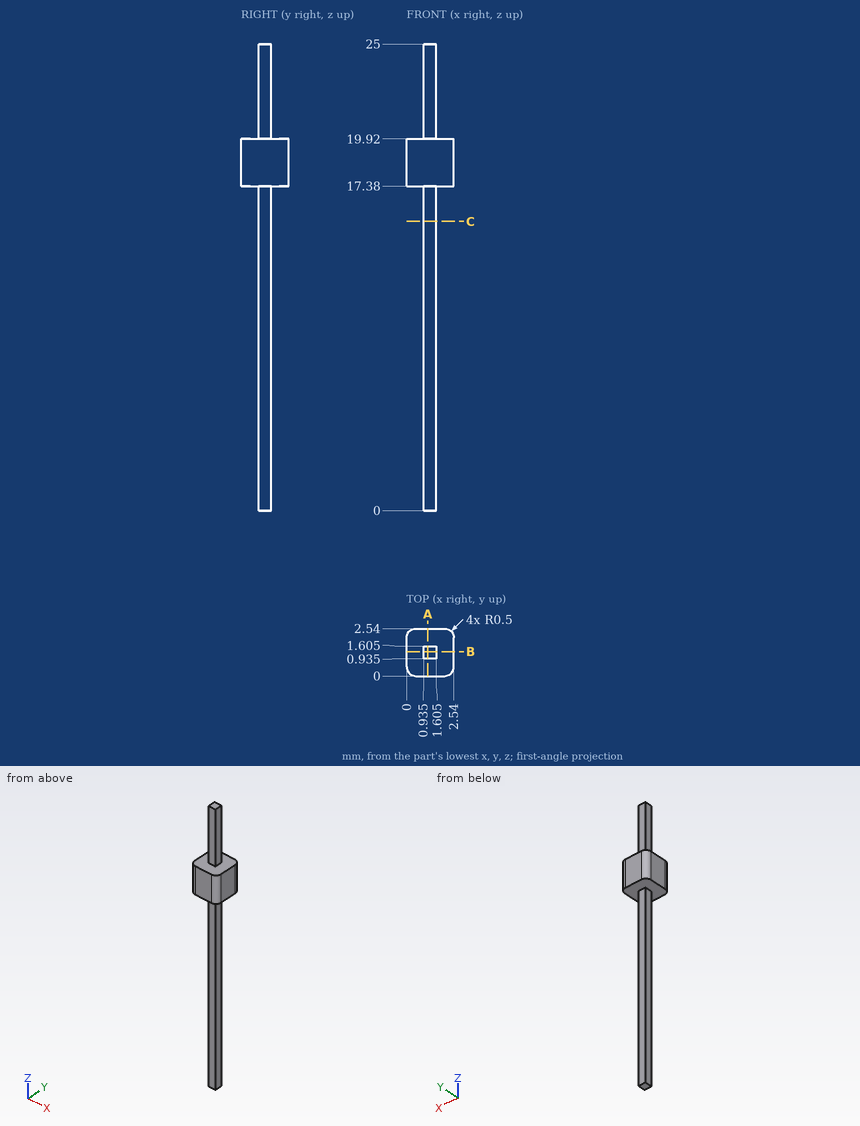
Geometry: see drawing. Coordinates: mm, zero at the bounding-box minimum. Coordinates: 2 decimals unless noted, no trailing zeros. Loops run counter-clockwise (first coordinate to the right, second up) from the corner with the lowest first, then second, coordinate; pieces in that order, holes last. Notation, with made-up numbers: M -14,49.5 L 22,49.5 A22 cw 22,67.5 Z; hole C 8,54.5 d7. An arc over 180 degrees is marked long. Put each result on its own line as item: value. Start each with the question number.
1) Cut plane C-C on z = 15.5. Return the cut outline in (x, y) (3 decimals), then the cut area to 3 significant figures.
2) Contact query for flat-ended pins moving along their axis: pin 1 Ø0.5 at (y, z) = (1.5, 7) entering from -X (3 decimals); pin 2 Ø0.5 at (y, z) = (1.5, 12) entering from +X (3 decimals); pin 3 Ø1 at (x, z) = (1, 5) entering from +Y (3 decimals). Output: stop coordinate, or through.
3) Ray query, L1, parallel to Y at x = 1.2, z = 21.5 (3 decimals); L2, parallel to Z at x = 1.1, y = 2.3. Return the intervals inside material, ascending. Write a range as from..to.
4) Cut plane A-A on x = 1.15. Return the cut outline in (y, z) (3 decimals).
The answers:
1. outline: M 0.935,0.935 L 1.605,0.935 L 1.605,1.605 L 0.935,1.605 Z
1. area: 0.449 mm²
2. pin 1: stops at x = 0.935
2. pin 2: stops at x = 1.605
2. pin 3: stops at y = 1.605
3. L1: y = 0.935..1.605
3. L2: z = 17.38..19.92
4. outline: M 0,17.38 L 0.935,17.38 L 0.935,0 L 1.605,0 L 1.605,17.38 L 2.54,17.38 L 2.54,19.92 L 1.605,19.92 L 1.605,25 L 0.935,25 L 0.935,19.92 L 0,19.92 Z
